The listing builds one solid part. Answer for the finished solid, in the listing's coordinates (mm). A direction names the side the tool comes from. Give positions to 0.01 mm unless a question says otherwise; leave off trailing zeros. Loops run counter-clockwise (first coordinate to the right, second up) from the corner with the lowest first, then second, coordinate; pieces in that order, holes last. Notation, with made-up numbers: (38.25, -20) - (45.25, -20) arc R4 ccw to (45.25, -13) - close; hole circle Ø10 at (-7, -4.75). An arc over 180 degrees is marked (long way). One line per item, written item: value. Start each with the question number.
from build123d import *

# Parameters (mm, degrees)
F0_W        = 120
F0_H        = 30
F1_DEPTH    = 20
F3_DEPTH    = 25
F4_DEPTH    = 5
F5_T1_DEPTH = 85
F5_T3_DEPTH = 145
F5_T5_DEPTH = 55


# Not quite as in the source:
# - a fillet or chamfer that OpenCascade refuses, or shapes differently, is made with other operations: its cross-section is extruded or revolved along the edge and cut away or added


with BuildPart() as f1:
    # F0 (on Top) → F1 (new body)
    with BuildSketch(Plane.XY):
        Rectangle(F0_W, F0_H)
    extrude(amount=F1_DEPTH)

    # F2 (on face) → F3 (cut)
    with BuildSketch(Plane.XY.offset(20)):
        Polygon((9, 11.5), (9, 0), (30, 0), (51, 0), (51, 11.5), align=None)
        Polygon((30, 0), (9, 0), (9, -11.5), (51, -11.5), (51, 0), align=None)
    extrude(amount=-F3_DEPTH, mode=Mode.SUBTRACT)

    # F2 (on face) → F4 (cut)
    with BuildSketch(Plane.XY.offset(20)):
        Polygon((0, 15), (0, 0), (9, 0), (9, 11.5), (51, 11.5), (51, 0), (60, 0), (60, 15), align=None)
        Polygon((9, 0), (0, 0), (0, -15), (60, -15), (60, 0), (51, 0), (51, -11.5), (9, -11.5), align=None)
    extrude(amount=-F4_DEPTH, mode=Mode.SUBTRACT)

    # F5: fillet of radius 5 on 7 edges, made by hand

    # F5_s2 → F5_t1 (cut)
    with BuildSketch(Plane.YZ.offset(-72.5)):
        with BuildLine():
            ThreePointArc((-15, 15), (-13.5355339059, 18.5355339059), (-10, 20))
            Line((-10, 20), (-15, 20))
            Line((-15, 20), (-15, 15))
        make_face()
        with BuildLine():
            ThreePointArc((15, 15), (13.5355339059, 18.5355339059), (10, 20))
            Line((10, 20), (15, 20))
            Line((15, 20), (15, 15))
        make_face()
    extrude(amount=F5_T1_DEPTH, mode=Mode.SUBTRACT)

    # F5_s4 → F5_t3 (cut)
    with BuildSketch(Plane.YZ.offset(-72.5)):
        with BuildLine():
            ThreePointArc((-10, 0), (-13.5355339059, 1.4644660941), (-15, 5))
            Line((-15, 5), (-15, 0))
            Line((-15, 0), (-10, 0))
        make_face()
        with BuildLine():
            ThreePointArc((10, 0), (13.5355339059, 1.4644660941), (15, 5))
            Line((15, 5), (15, 0))
            Line((15, 0), (10, 0))
        make_face()
    extrude(amount=F5_T3_DEPTH, mode=Mode.SUBTRACT)

    # F5_s6 → F5_t5 (cut)
    with BuildSketch(Plane.XZ.offset(-27.5)):
        with BuildLine():
            ThreePointArc((60, 5), (58.5355339059, 1.4644660941), (55, 0))
            Line((55, 0), (60, 0))
            Line((60, 0), (60, 5))
        make_face()
        with BuildLine():
            ThreePointArc((-55, 0), (-58.5355339059, 1.4644660941), (-60, 5))
            Line((-60, 5), (-60, 0))
            Line((-60, 0), (-55, 0))
        make_face()
        with BuildLine():
            ThreePointArc((-60, 15), (-58.5355339059, 18.5355339059), (-55, 20))
            Line((-55, 20), (-60, 20))
            Line((-60, 20), (-60, 15))
        make_face()
    extrude(amount=F5_T5_DEPTH, mode=Mode.SUBTRACT)


solid = f1.part
1. For faces 4 (the flat face through (30, -13, 15)), 5 (the flat face through (-1, -15, 10)), 6 (the flat face through (9, 0, 8)), determine the directions among +Z, -Z, +X, -X, +Y, -Y from which every point of the face is accessible in a straight line to the end or side of a thin tool.
2. Flat-ended cylindrical pins translate along their axes: pin 1 (5 mm diameter, centred on x = -35, z = 2.5, fed in from -Y); pin 2 (5.5 mm diameter, centred on y = -4, z = 18.5, fed in from +X); pin 3 (1 mm diameter, centred on x = -17, z = 3, fed in from +Y); pin 4 (6 mm diameter, centred on x = 4.5, y = -4, fed in from +Z). Find the tip coordinate at first contact, or state that the pin passes through.
3. A cutting plane is placed at B-B (x = 47.5). Determine the outline of the cut face in (y, z), plus the area to 3 significant figures.
4. Determine the mould class of faces 1 (the flat face through (30, 11.5, 8)), 2 (the flat face through (60, 0, 10)), 3 (the flat face through (-28, 0, 20)) for opening direction X: released by +X, released by -X, zero draft, split by the parting line, or undercut.
5. A cutting plane is placed at A-A (z = 12). Determine the outline of the cut face in (x, y), plus the area to 3 significant figures.
6. A cutting plane is placed at D-D (x = -14). Determine the outline of the cut face in (y, z).
7. A cutting plane is placed at C-C (y = -0.5). Determine the outline of the cut face in (x, z), plus the area to 3 significant figures.
8. Find the intervals of material crossed by L1, parallel to X at y = 7, z = 6; L2, parallel to Y at x = 17.5, z = 7.5; L3, parallel to Z at x = 52.5, y = 4.75, in increasing order. Write a range as [from, to].
Results below:
1. face 4: +Z, +X, +Y, -Y
1. face 5: +Z, -Z, +X, -X, -Y
1. face 6: +Z, -Z
2. pin 1: stops at y = -15
2. pin 2: stops at x = 0
2. pin 3: stops at y = 14.77
2. pin 4: stops at z = 15
3. outline: (-15, 5) arc R5 ccw to (-11.5, 0.23) - (-11.5, 15) - (-15, 15) - close; (11.5, 0.23) arc R5 ccw to (15, 5) - (15, 15) - (11.5, 15) - close
3. area: 94.5 mm^2
4. face 1: undercut
4. face 2: released by +X
4. face 3: zero draft
5. outline: (-60, -15) - (60, -15) - (60, 15) - (-60, 15) - close; hole (9, -11.5) - (51, -11.5) - (51, 11.5) - (9, 11.5) - close
5. area: 2,630 mm^2
6. outline: (-15, 5) arc R5 ccw to (-10, 0) - (10, 0) arc R5 ccw to (15, 5) - (15, 15) arc R5 ccw to (10, 20) - (-10, 20) arc R5 ccw to (-15, 15) - close
7. outline: (-60, 5) arc R5 ccw to (-55, 0) - (9, 0) - (9, 15) - (0, 15) - (0, 20) - (-55, 20) arc R5 ccw to (-60, 15) - close; (51, 0) - (55, 0) arc R5 ccw to (60, 5) - (60, 15) - (51, 15) - close
7. area: 1,450 mm^2
8. L1: x = [-60, 9], [51, 60]
8. L2: y = [-15, -11.5], [11.5, 15]
8. L3: z = [0, 15]
